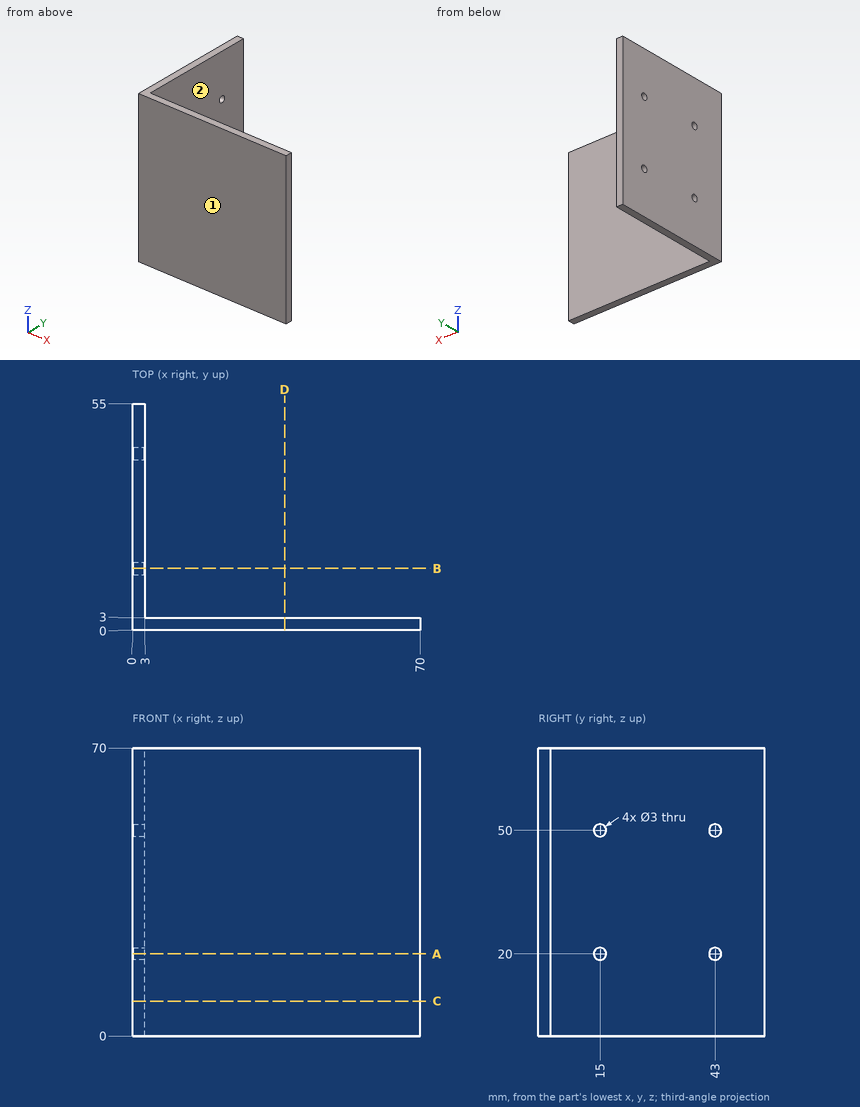
The drawing under review shows one solid part. Ordinate dimensions are in mm from its lowest x, y, z. A direction names the side the tool comes from. Coordinates: 2 decimals unless noted, no trailing zeros. Write each loop counter-clockwise with the first axis right and the second up, starting at its lowest first coordinate (ties: lowest second). Pieces come first, ordered by that corner, then holes. Notation, with made-up numbers: (24, -19.75) - (37, -19.75) arc R22 ccw to (37, 13.25) - close; hole circle Ø7 at (33.5, -11). An arc over 180 degrees is marked (long way). Put each result on its own line as item: value.
1. Machinability: for the marked faces 1 and 2, which of the approach directions +Z, -Z, +X, -X, +Y, -Y give a long, thin tool a straight path to every point of the face, cutting with its end or side? Answer none if there is none.
Values found:
face 1: +Z, -Z, +X, -X, -Y
face 2: +Z, -Z, +X, +Y
2. Add section B-B, the plane y = 15. Give the boundary of the cut face in (x, z), then the cut area to 3 significant figures.
Values found:
outline: (0, 0) - (3, 0) - (3, 18.5) - (0, 18.5) - close; (0, 21.5) - (3, 21.5) - (3, 48.5) - (0, 48.5) - close; (0, 51.5) - (3, 51.5) - (3, 70) - (0, 70) - close
area: 192 mm²
3. For pin 1 (1.5 mm diameter, centred on y = 8.5, z = 32.5, fed in from +X); pin 2 (8 mm diameter, centred on x = 24.5, z = 46, fed in from -Y); pin 3 (3 mm diameter, centred on x = 44, z = 45.5, fed in from +Y), all flat-tipped, find the tip position at first contact; note any pin that passes through.
Values found:
pin 1: x = 3
pin 2: y = 0
pin 3: y = 3
4. Wall thickness on probe 1 along Y at (x, z) = (1.35, 50); probe 2 along X at (y, z) = (37.5, 59.5): over which ranges is each line inside the solid? List them lowest first.
Values found:
probe 1: 0 to 13.5, 16.5 to 41.5, 44.5 to 55
probe 2: 0 to 3
5. Add section C-C, the plane z = 8.5. Give the boundary of the cut face in (x, y).
Values found:
outline: (0, 0) - (70, 0) - (70, 3) - (3, 3) - (3, 55) - (0, 55) - close
6. Add section D-D, the plane x = 37. Give the boundary of the cut face in (y, z).
Values found:
outline: (0, 0) - (3, 0) - (3, 70) - (0, 70) - close
7. Add section A-A, the plane z = 20. Give the boundary of the cut face in (x, y).
Values found:
outline: (0, 0) - (70, 0) - (70, 3) - (3, 3) - (3, 13.5) - (0, 13.5) - close; (0, 16.5) - (3, 16.5) - (3, 41.5) - (0, 41.5) - close; (0, 44.5) - (3, 44.5) - (3, 55) - (0, 55) - close
